The listing builds one solid part. Answer for the finished solid, in the listing's coordinates (mm). Face numbers are marked on the shaded views. A direction names the side the tool comes from. Coordinates: 2 decimals unless noted, no trailing zeros. Order: outer loops, then holes, each group sorted by start corner. A loop starts at its lowest first (then second) coordinate and runs counter-clockwise, first axis right, second up. Notation, with made-up numbers: (-16.75, 75.25) -> (3.25, 75.25) arc R30 ccw to (3.25, 113.25) -> close; hole circle Ø9 at (31.5, 84.25). An arc over 180 degrees is marked (long way). Return JSON: item names as keys, results as strings.
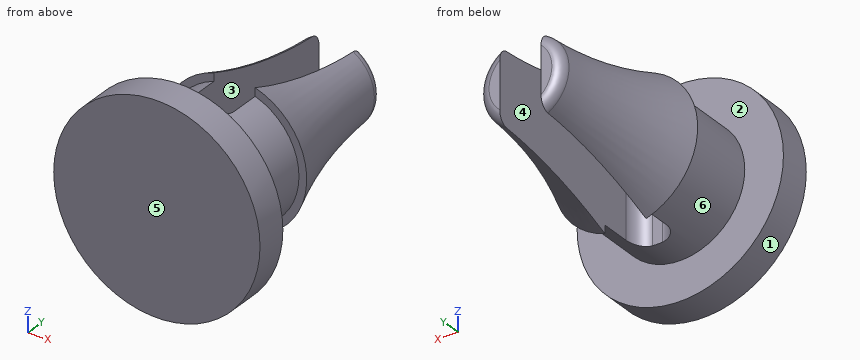
```python
from build123d import *

# Parameters (mm, degrees)
CUT_EXTRUDE1_DEPTH      = 15.591189122
CUT_EXTRUDE1_DEPTH_BACK = 15.591189122


with BuildPart() as part:
    # Sketch1 → Revolve1 (revolve)
    with BuildSketch(Plane.XY):
        with BuildLine():
            Line((0, 0), (-5.08, 0))
            Line((-5.08, 0), (-5.08, 1.5875))
            Line((-5.08, 1.5875), (-3.175, 1.5875))
            Line((-3.175, 1.5875), (-3.175, 5.3975))
            Line((-3.175, 5.3975), (-3.556, 5.3975))
            ThreePointArc((-3.556, 5.3975), (-2.52664009, 8.747354796), (-2.052787845, 12.219612423))
            ThreePointArc((-2.052787845, 12.219612423), (-1.894850225, 12.560843538), (-1.545538839, 12.7))
            Line((-1.545538839, 12.7), (0, 12.7))
            Line((0, 12.7), (0, 0))
        make_face()
    revolve(axis=Axis((0, 12.7, 0), (0, -1, 0)))

    # Sketch2 → Cut-Extrude1 (cut, two sides: drawn at the far end of the back side and taken through both)
    with BuildSketch(Plane.XY.offset(-CUT_EXTRUDE1_DEPTH_BACK)):
        with BuildLine():
            Line((-0.254, 3.175), (0.254, 3.175))
            ThreePointArc((0.254, 3.175), (0.792815367, 3.398184633), (1.016, 3.937))
            Line((1.016, 3.937), (1.016, 12.7))
            Line((1.016, 12.7), (-1.016, 12.7))
            Line((-1.016, 12.7), (-1.016, 3.937))
            ThreePointArc((-1.016, 3.937), (-0.792815367, 3.398184633), (-0.254, 3.175))
        make_face()
    extrude(amount=CUT_EXTRUDE1_DEPTH + CUT_EXTRUDE1_DEPTH_BACK, mode=Mode.SUBTRACT)


solid = part.part
```
Item 1: The part is cut by section A-A on x = 0. Determine the outline of the cut face in (y, z) (1 decimal).
Answer list:
{"outline": "(0, -5.1) -> (1.6, -5.1) -> (1.6, -3.2) -> (3.2, -3.2) -> (3.2, 3.2) -> (1.6, 3.2) -> (1.6, 5.1) -> (0, 5.1) -> close"}
Item 2: Determine the mould class of the marked faces 1, 2, 3 and 4 for opening direction X: pulls with the +X half, pulls with the -X half, needs draft (parallel to the pull), parting line crosses it, or undercut.
Answer list:
{"face 1": "parting line crosses it", "face 2": "needs draft", "face 3": "undercut", "face 4": "undercut"}
Item 3: Flat-ended cylindrical pins translate along their axes: pin 1 (3 mm diameter, centred on x = -2, z = -1, fed in from -Y); pin 2 (1.5 mm diameter, centred on y = 3, z = 1, fed in from +X); pin 3 (5 mm diameter, centred on y = 7, z = -0.5, fed in from +X); pin 4 (3.5 mm diameter, centred on y = 8.5, z = 1.5, fed in from +X). Find the tip coordinate at first contact, or state that the pin passes through.
Answer list:
{"pin 1": "y = 0", "pin 2": "x = 3.17", "pin 3": "x = 3.56", "pin 4": "x = 2.93"}
Item 4: The part is cut by section C-C on y = 9.25. Determine the outline of the cut face in (x, z).
Answer list:
{"outline": "(-1.02, -2.2) -> (-1.02, 2.2) arc R2.42 ccw to start; (1.02, -2.2) arc R2.42 ccw to (1.02, 2.2) -> close"}
Item 5: The part is cut by section D-D on y = 4.5. Determine the outline of the cut face in (x, z) (3 decimals), plus the area to 3 significant figures.
Answer list:
{"outline": "(-1.016, -3.008) -> (-1.016, 3.008) arc R3.175 ccw to start; (1.016, -3.008) arc R3.175 ccw to (1.016, 3.008) -> close", "area": "19.0 mm2"}
Item 6: Which of the six approach directions +Z, -Z, +X, -X, +Y, -Y give full straight-line access (tool end or side, diameter ignored) to the marked faces 5 and 6?
Answer list:
{"face 5": "+Z, -Z, +X, -X, -Y", "face 6": "none"}
Item 7: Find the intervals of material crossed by probe 1 along X at (y, z) = (7.25, 1); probe 2 along X at (y, z) = (4.5, 2.5); probe 3 along Y at (x, z) = (4, -3), in increasing order.
Answer list:
{"probe 1": "-2.74 to -1.02, 1.02 to 2.74", "probe 2": "-1.96 to -1.02, 1.02 to 1.96", "probe 3": "0 to 1.59"}
